Read the model definition and answer for the solid it produces. Units are mm, in the model's axes. A direction names the side the tool comes from. Coordinates: 2 decimals unless noted, no trailing zeros. Order: outer loops, then holes, each group sorted by start corner. A loop starts at its lowest first (then second) coordinate and runs counter-clockwise, first axis right, second up. Notation, with made-up numbers: (27, -38.5) - (65, -38.5) arc R23 cw to (65, -15.5) - close; hole circle Ø6 at (-9.5, -13). An arc over 180 degrees is marked (long way). Use one line per item in the form item = value. Start each with the question number.
from build123d import *

# Parameters (mm, degrees)
SKETCH2_R           = 1.4
BOSS_EXTRUDE1_DEPTH = 2


with BuildPart() as part:
    # Sketch2 → Boss-Extrude1 (new body)
    with BuildSketch(Plane.XY):
        Polygon((0, 0), (0, 53.34), (66, 53.34), (66, 40.54), (68.54, 37.473610341), (68.54, 4.765453974), (66, 1.699064314), (66, 0), align=None)
        with Locations((15.24, 50.8)):
            Circle(SKETCH2_R, mode=Mode.SUBTRACT)
        with Locations((66, 35.56)):
            Circle(SKETCH2_R, mode=Mode.SUBTRACT)
        with Locations((66, 7.62)):
            Circle(SKETCH2_R, mode=Mode.SUBTRACT)
    extrude(amount=-BOSS_EXTRUDE1_DEPTH)


solid = part.part
Q1. Consider probe 1 along X at (y, z) = (42, -0.25); probe 2 along X at (y, z) = (4.5, -0.9). Determine where each line is inside the solid, lowest interval first.
Q2. A cutting plane is placed at C-C (z = -0.4). Give the vertices of the cut face in (x, y), then the cut area to 3 significant figures.
Q3. A cutting plane is placed at A-A (x = 15.24). Give the vertices of the cut face in (y, z), then the cut area to 3 significant figures.
Q4. A cutting plane is placed at B-B (y = 35.56). Give the vertices of the cut face in (x, z).
Q5. A cutting plane is placed at D-D (y = 44.5). Give the vertices of the cut face in (x, z), then the cut area to 3 significant figures.
Q6. Which of the six approach directions +Z, -Z, +X, -X, +Y, -Y give full straight-line access (tool end or side, diameter ignored) to faces 1 (the flat face through (33, 0, -1)), 2 (the flat face through (66, 1, -1))?
Q7. Given P1, Ø0.8, axis at y = 0.5, z = -0.5, coming from the +X side, flat-ended and moving along its own axis, determine where the tip first touches the part or whether it passes through.
Q8. For a pull along X with two mould halves and no side action, classify faces 3 (the flat face through (0, 26, -1)), 4 (the flat face through (66, 47, -1)), 5 (the cylindrical face through (66.75, 36.74, -0.99)), 6 (the flat face through (35, 27, -2)) as +X half, -X half, draft (parallel to the pull), parting line (faces both ways), or undercut.
Result sheet:
q1.probe_1 = 0 to 66
q1.probe_2 = 0 to 68.32
q2.outline = (0, 0) - (66, 0) - (66, 1.7) - (68.54, 4.77) - (68.54, 37.47) - (66, 40.54) - (66, 53.34) - (0, 53.34) - close; hole circle Ø2.8 at (15.24, 50.8); hole circle Ø2.8 at (66, 7.62); hole circle Ø2.8 at (66, 35.56)
q2.area = 3,590 mm^2
q3.outline = (0, -2) - (49.4, -2) - (49.4, 0) - (0, 0) - close; (52.2, -2) - (53.34, -2) - (53.34, 0) - (52.2, 0) - close
q3.area = 101 mm^2
q4.outline = (0, -2) - (64.6, -2) - (64.6, 0) - (0, 0) - close; (67.4, -2) - (68.54, -2) - (68.54, 0) - (67.4, 0) - close
q5.outline = (0, -2) - (66, -2) - (66, 0) - (0, 0) - close
q5.area = 132 mm^2
q6.face_1 = +Z, -Z, +X, -X, -Y
q6.face_2 = +Z, -Z, +X, -Y
q7.P1 = 66
q8.face_3 = -X half
q8.face_4 = +X half
q8.face_5 = undercut
q8.face_6 = draft
